Check sheet for the modelled part. Datum: model origin and axes. Units: mm. A direction names the side the tool comes from. Round coordinates to 2 decimals unless told otherwise and drop trailing zeros. Write each loop counter-clockwise with the first axis right and the second up, starting at its lowest first coordinate (ties: lowest second). Pieces come first, ordered by that corner, then holes. Notation, with made-up numbers: (66, 5) -> (80, 5) arc R21 ccw to (80, 32) -> close; hole circle Ø5 at (63.5, 76). An arc over 180 degrees is marked (long way). One line per item, written item: value. Start each with the question number.
Autodesk Inventor part; units mm, degrees
ref_plane "YZ Plane" through (0, 0, 0) normal (1, 0, 0) x (0, 1, 0)
ref_plane "XZ Plane" through (0, 0, 0) normal (0, 1, 0) x (-1, 0, 0)
ref_plane "XY Plane" through (0, 0, 0) normal (0, 0, 1) x (1, 0, 0)
ref_plane "Work Plane1" through (0, 0, 0) normal (0, 0, 1) x (1, 0, 0)
sketch "Sketch1" plane through (0, 0, 0) normal (0, 0, 1) x (1, 0, 0)
  line L0 (247.5, -5.2779) -> (147.5, -5.2779)
  line L1 (147.5, -5.2779) -> (147.5, 14.7221)
  line L2 (147.5, 14.7221) -> (247.5, 14.7221)
  line L3 (247.5, 14.7221) -> (247.5, -5.2779)
  line L4 (235, 40.7039) -> (235, 15.7039)
  line L5 (160, 15.7039) -> (160, 40.7039)
  line L6 (161, 181.7039) -> (234, 181.7039)
  arc A0 (235, 180.7039) -> (234, 181.7039) centre (234, 180.7039) ccw
  line L7 (235, 180.7039) -> (235, 155.7039)
  arc A1 (234, 154.7039) -> (235, 155.7039) centre (234, 155.7039) ccw
  line L8 (234, 154.7039) -> (219.9889, 154.7039)
  line L9 (219.9889, 154.7039) -> (219.9889, 41.7039)
  line L10 (219.9889, 41.7039) -> (234, 41.7039)
  arc A2 (235, 40.7039) -> (234, 41.7039) centre (234, 40.7039) ccw
  line L11 (235, 40.7039) -> (235, 15.7039)
  arc A3 (234, 14.7039) -> (235, 15.7039) centre (234, 15.7039) ccw
  line L12 (234, 14.7039) -> (229.5826, 14.7039)
  line L13 (229.5826, 14.7039) -> (229.5826, 21.7039)
  line L14 (229.5826, 21.7039) -> (220.4174, 21.7039)
  line L15 (220.4174, 21.7039) -> (220.4174, 14.7039)
  line L16 (220.4174, 14.7039) -> (174.5826, 14.7039)
  line L17 (174.5826, 14.7039) -> (174.5826, 21.7039)
  line L18 (174.5826, 21.7039) -> (165.4174, 21.7039)
  line L19 (165.4174, 21.7039) -> (165.4174, 14.7039)
  line L20 (165.4174, 14.7039) -> (161, 14.7039)
  arc A4 (160, 15.7039) -> (161, 14.7039) centre (161, 15.7039) ccw
  line L21 (160, 15.7039) -> (160, 40.7039)
  arc A5 (161, 41.7039) -> (160, 40.7039) centre (161, 40.7039) ccw
  line L22 (161, 41.7039) -> (175.0111, 41.7039)
  line L23 (175.0111, 41.7039) -> (175.0111, 154.7039)
  line L24 (175.0111, 154.7039) -> (161, 154.7039)
  arc A6 (160, 155.7039) -> (161, 154.7039) centre (161, 155.7039) ccw
  line L25 (160, 155.7039) -> (160, 180.7039)
  arc A7 (161, 181.7039) -> (160, 180.7039) centre (161, 180.7039) ccw
  line L26 (161, 181.7039) -> (234, 181.7039)
  arc A8 (235, 180.7039) -> (234, 181.7039) centre (234, 180.7039) ccw
  line L27 (235, 180.7039) -> (235, 155.7039)
  arc A9 (234, 154.7039) -> (235, 155.7039) centre (234, 155.7039) ccw
  line L28 (234, 154.7039) -> (219.9889, 154.7039)
  line L29 (219.9889, 154.7039) -> (219.9889, 41.7039)
  line L30 (219.9889, 41.7039) -> (234, 41.7039)
  arc A10 (235, 40.7039) -> (234, 41.7039) centre (234, 40.7039) ccw
  line L31 (235, 40.7039) -> (235, 15.7039)
  arc A11 (234, 14.7039) -> (235, 15.7039) centre (234, 15.7039) ccw
  line L32 (234, 14.7039) -> (229.5826, 14.7039)
  line L33 (229.5826, 14.7039) -> (229.5826, 21.7039)
  line L34 (229.5826, 21.7039) -> (220.4174, 21.7039)
  line L35 (220.4174, 21.7039) -> (220.4174, 14.7039)
  line L36 (220.4174, 14.7039) -> (174.5826, 14.7039)
  line L37 (174.5826, 14.7039) -> (174.5826, 21.7039)
  line L38 (174.5826, 21.7039) -> (165.4174, 21.7039)
  line L39 (165.4174, 21.7039) -> (165.4174, 14.7039)
  line L40 (165.4174, 14.7039) -> (161, 14.7039)
  arc A12 (160, 15.7039) -> (161, 14.7039) centre (161, 15.7039) ccw
  line L41 (160, 15.7039) -> (160, 40.7039)
  arc A13 (161, 41.7039) -> (160, 40.7039) centre (161, 40.7039) ccw
  line L42 (161, 41.7039) -> (175.0111, 41.7039)
  line L43 (175.0111, 41.7039) -> (175.0111, 154.7039)
  line L44 (175.0111, 154.7039) -> (161, 154.7039)
  arc A14 (160, 155.7039) -> (161, 154.7039) centre (161, 155.7039) ccw
  line L45 (160, 155.7039) -> (160, 180.7039)
  arc A15 (161, 181.7039) -> (160, 180.7039) centre (161, 180.7039) ccw
  line L46 (0, 0) -> (400, 0)
  line L47 (400, 0) -> (400, -5.0961)
  line L48 (0, -5.0961) -> (400, -5.0961)
  line L49 (0, -5.0961) -> (0, 0)
  line L50 (0, 14.5039) -> (400, 14.5039)
  line L51 (400, 14.5039) -> (400, 9.6864)
  line L52 (400, 9.6864) -> (0, 9.6864)
  line L53 (0, 9.6864) -> (0, 14.5039)
  circle A16 centre (240, 4.7221) radius 2.6
  circle A17 centre (155, 4.7221) radius 2.6
  point P0 (153.6248, 9.6864)
  point P1 (156.3752, 9.6864)
  point P2 (241.3752, 9.6864)
  point P3 (238.6248, 9.6864)
  dimension "d1" = 100
  dimension "d4" = -12.5
  dimension "d5" = 12.5
  dimension "d6" = 5.2
  dimension "d7" = 5.2
  dimension "d8" = 7.5
  dimension "d9" = 7.5
  dimension "d22" = 20
  dimension "d23" = 10
  dimension "d24" = 10
extrude "Extrusion1" add sketch "Sketch1" along normal blind 5.3 contours L0 L1 L48 L3 | L48 L1 L46 L3 | L46 L1 L52 L3 | L52 L1 L50 L3 | L50 L1 L2 A4 L20 L19 L17 L16 L15 L13 L12 A3 L3 | A3 L12 L13 L2 | L2 L19 L20 A4 | L15 L16 L17 L2
sketch "Sketch2" plane through (147.5, -5.2779, 0) normal (0, -1, 0) x (1, 0, 0)
  circle A0 centre (50, 25.5) radius 19
  line L0 (69, 25.5) -> (84, 25.5)
  line L1 (31, 25.5) -> (16, 25.5)
  line L2 (16, 25.5) -> (16, 5.3)
  line L3 (0, 5.3) -> (100, 5.3)
  line L4 (84, 25.5) -> (84, 5.3)
  line L5 (84, 24.5) -> (68.9737, 24.5)
  line L6 (31.0263, 24.5) -> (16, 24.5)
  point P0 (-147.5, 0)
  dimension "d10" = 15
  dimension "d11" = 15
  dimension "d14" = 1
extrude "Extrusion2" add sketch "Sketch2" against normal up to surface (20 mm away) contours L5 L4 L3 L2 L6 A0
sketch "Sketch3" plane through (216.4737, -5.2779, 24.5) normal (0, 0, 1) x (1, 0, 0)
  circle A0 centre (7.5263, 10) radius 3
  circle A1 centre (-45.4737, 10) radius 3
  line L0 (15.0263, 0) -> (15.0263, 20)
  line L1 (0, 0) -> (0, 20)
  line L2 (-52.9737, 0) -> (-52.9737, 20)
  line L3 (-37.9473, 0) -> (-52.9737, 0)
  line L4 (15.0263, 0) -> (0, 0)
  point P0 (-216.4737, 5.2779)
  point P1 (15.0263, 10)
  dimension "d15" = 6
  dimension "d16" = 6
  dimension "d17" = 7.5
  dimension "d19" = 7.5
  dimension "d25" = 10
  dimension "d26" = 10
extrude "Extrusion3" cut sketch "Sketch3" against normal blind 17
sketch "Sketch4" plane through (147.5, -5.2779, 0) normal (0, -1, 0) x (1, 0, 0)
  line L0 (84, 24.5) -> (68.9737, 24.5)
  line L1 (84, 24.5) -> (16, 24.5)
  line L2 (16, 24.5) -> (16, 5.3)
  line L3 (16, 5.3) -> (84, 5.3)
  line L4 (84, 5.3) -> (84, 24.5)
  arc A0 (31.0263, 24.5) -> (68.9737, 24.5) centre (50, 25.5) ccw
  circle A1 centre (50, 25.5) radius 12.5
  point P0 (-147.5, 0)
  point P1 (62.4599, 24.5)
  point P2 (37.5401, 24.5)
  dimension "d27" = 25
extrude "Extrusion4" add sketch "Sketch4" against normal blind 4 contours L4 L3 L2 L1 A0 L0 | A0 L1 A1
sketch "Sketch5" plane through (147.5, -5.2779, 0) normal (0, -1, 0) x (1, 0, 0)
  line L0 (81, 16.5) -> (72, 16.5)
  line L1 (72, 16.5) -> (72, 11.5)
  line L2 (72, 11.5) -> (81, 11.5)
  line L3 (81, 11.5) -> (81, 16.5)
  line L4 (73.5, 24.5) -> (79.5, 24.5)
  line L5 (20.5, 24.5) -> (26.5, 24.5)
  line L6 (20.5, 7.5) -> (26.5, 7.5)
  line L7 (20.5, 24.5) -> (26.5, 24.5)
  line L8 (73.5, 7.5) -> (79.5, 7.5)
  line L9 (73.5, 24.5) -> (79.5, 24.5)
  line L10 (28, 16.5) -> (19, 16.5)
  line L11 (19, 16.5) -> (19, 11.5)
  line L12 (19, 11.5) -> (28, 11.5)
  line L13 (28, 11.5) -> (28, 16.5)
  point P0 (-147.5, 0)
  point P1 (76.5, 24.5)
  point P2 (76.5, 16.5)
  point P3 (23.5, 24.5)
  point P4 (23.5, 16.5)
  dimension "d30" = 9
  dimension "d31" = 5
  dimension "d32" = 6
  dimension "d33" = 1.5
  dimension "d34" = 8
  dimension "d35" = 9
  dimension "d36" = 5
  dimension "d37" = 6
  dimension "d38" = 1.5
  dimension "d39" = 8
extrude "Extrusion5" cut sketch "Sketch5" against normal blind 15
sketch "Sketch6" plane through (147.5, 14.7221, 0) normal (0, 1, 0) x (1, 0, 0)
  line L0 (81, -11.5) -> (72, -11.5)
  line L1 (72, -11.5) -> (72, -16.5)
  line L2 (72, -16.5) -> (81, -16.5)
  line L3 (81, -16.5) -> (81, -11.5)
  line L4 (28, -11.5) -> (19, -11.5)
  line L5 (19, -11.5) -> (19, -16.5)
  line L6 (19, -16.5) -> (28, -16.5)
  line L7 (28, -16.5) -> (28, -11.5)
  line L8 (0, -5.3) -> (16, -5.3)
  line L9 (0, 0) -> (0, -5.3)
  line L10 (0, 0) -> (100, 0)
  line L11 (100, 0) -> (100, -5.3)
  line L12 (84, -5.3) -> (100, -5.3)
  line L13 (84, -5.3) -> (84, -24.5)
  line L14 (84, -24.5) -> (62.4599, -24.5)
  arc A0 (62.4599, -24.5) -> (37.5401, -24.5) centre (50, -25.5) ccw
  line L15 (37.5401, -24.5) -> (16, -24.5)
  line L16 (16, -24.5) -> (16, -5.3)
  line L17 (20.5, -11.5) -> (26.5, -11.5)
  line L18 (22, -11.5) -> (24, -11.5)
  line L19 (24, -11.5) -> (24, -16.5)
  line L20 (24, -16.5) -> (22, -16.5)
  line L21 (22, -16.5) -> (22, -11.5)
  line L22 (73.5, -11.5) -> (79.5, -11.5)
  line L23 (72, -16.5) -> (81, -16.5)
  line L24 (75, -11.5) -> (77, -11.5)
  line L25 (77, -11.5) -> (77, -16.5)
  line L26 (77, -16.5) -> (75, -16.5)
  line L27 (75, -16.5) -> (75, -11.5)
  point P0 (-147.5, 0)
  point P1 (22, -11.5)
  dimension "d42" = 2
  dimension "d43" = 9
  dimension "d44" = 3
  dimension "d45" = 2
  dimension "d46" = 3
extrude "Extrusion6" cut sketch "Sketch6" against normal through all contours L25 L2 L27 L0 | L19 L6 L21 L4
sketch "Sketch7" plane through (0, 0, 5.3) normal (0, 0, 1) x (1, 0, 0)
  circle A0 centre (240, 4.7221) radius 2.6
  circle A1 centre (240, 4.7221) radius 5.75
  circle A2 centre (155, 4.7221) radius 2.6
  circle A3 centre (155, 4.7221) radius 5.75
  point P0 (0, 0)
  dimension "d49" = 11.5
  dimension "d50" = 11.5
extrude "Extrusion7" cut sketch "Sketch7" against normal blind 2
equation "\"d30\" = d35"
equation "\"d31\" = d36"
equation "\"d33\" = -0.5 * d32 + 0.5 * d30"
equation "\"d38\" = -0.5 * d37 + 0.5 * d35"
equation "\"d49\" = d50"
properties part number "FrontPistonSupportButtom"
1. Access from +Z, -Z, +X, -X, +Y, -Y to the whole of each face (thin tool, end or side, straight path). Record for faces 5 (the face through (234, 5, 5.3)), 6 (the face through (173.861, 5.623, 20.556)), 7 (the face through (173, 9.722, 14)), 8 (the face through (197, -1.278, 12)).
2. Cross-section at D-D (x = 197.5). Record the cut outline in (y, z).
3. Depth check by flat-ended pin: pin 1 Ø9 at (x, y) = (154, 7) entering from +Z; pin 2 Ø2.5 at (x, z) = (168, 14) entering from -Y; pin 3 Ø5 at (y, z) = (12.5, 10.5) entering from +X. Enter the tip coordinate at first touch or a pass-through.
4. Release check for a two-part mould opening along Z. For faces 1 (the face through (221, 9.722, 14)), 2 (the face through (198, -5.278, 9)), 3 (the face through (219.5, 2, 14)), 4 (the face through (197.096, 6.61, 6.504)) record: +Z half, -Z half, draft (parallel to the pull), parting line (faces both ways), or undercut.
5. Material ranges on probe 1 along X at (y, z) = (-2.5, 12.75); probe 2 along Y at (x, z) = (224, 18.75); probe 3 along X at (y, z) = (7.75, 12.75), recorded low to high.
6. Cross-section at A-A (x = 240). Record the cut outline in (y, z), plus the area to 3 significant figures.
7. Cross-section at B-B (z = 20.25). Record the cut outline in (x, y).
8. Cross-section at C-C (y = -3.5). Record the cut outline in (x, z).
Working result:
1. face 5: +Z, +X, +Y, -Y
1. face 6: +Z
1. face 7: -Y
1. face 8: +Z, +Y
2. outline: (-5.28, 0) -> (14.72, 0) -> (14.72, 6.5) -> (-1.28, 6.5) -> (-1.28, 13) -> (-5.28, 13) -> close
3. pin 1: stops at z = 5.3
3. pin 2: stops at y = 9.72
3. pin 3: stops at x = 231.5
4. face 1: undercut
4. face 2: draft
4. face 3: undercut
4. face 4: +Z half
5. probe 1: x = 163.5 to 166.5, 175.5 to 219.5, 228.5 to 231.5
5. probe 2: y = -5.28 to 1.72, 7.72 to 14.72
5. probe 3: x = 163.5 to 166.5, 175.5 to 183.41, 211.59 to 219.5, 228.5 to 231.5
6. outline: (-5.28, 0) -> (2.12, 0) -> (2.12, 3.3) -> (-1.03, 3.3) -> (-1.03, 5.3) -> (-5.28, 5.3) -> close; (7.32, 0) -> (14.72, 0) -> (14.72, 5.3) -> (10.47, 5.3) -> (10.47, 3.3) -> (7.32, 3.3) -> close
6. area: 65.8 mm^2
7. outline: (163.5, -5.28) -> (186.16, -5.28) -> (186.16, -1.28) -> (179.24, -1.28) -> (179.24, 14.72) -> (163.5, 14.72) -> close; (208.84, -5.28) -> (231.5, -5.28) -> (231.5, 14.72) -> (215.76, 14.72) -> (215.76, -1.28) -> (208.84, -1.28) -> close; hole circle Ø6 at (171, 4.72); hole circle Ø6 at (224, 4.72)
8. outline: (147.5, 0) -> (247.5, 0) -> (247.5, 5.3) -> (231.5, 5.3) -> (231.5, 24.5) -> (209.96, 24.5) arc R12.5 cw to (185.04, 24.5) -> (163.5, 24.5) -> (163.5, 5.3) -> (147.5, 5.3) -> close; hole (166.5, 11.5) -> (175.5, 11.5) -> (175.5, 16.5) -> (166.5, 16.5) -> close; hole (219.5, 11.5) -> (228.5, 11.5) -> (228.5, 16.5) -> (219.5, 16.5) -> close
